Geometry: final body of the model. Coordinates: model frame, mm. Face numbers are marked on the shaded views. Round coordinates to 2 decimals unless told otherwise and drop trailing zeros. Order: outer loops, then holes, each group sorted by start corner. A loop starts at its lowest first (then second) coordinate and runs counter-clockwise, first axis right, second up. Notation, with made-up numbers: (64.5, 14.25) - (93.5, 14.25) arc R19 ccw to (93.5, 37.25) - close; hole circle Ø4 at (31, 22.5). An arc over 180 degrees is marked (long way). Put each result on its own line as item: value. Start each with the question number.
(1) Section C-C (z = 0). Output: boundary loops of the cut face in (x, y) (1 decimal), and give its area (3 significant figures).
(2) Pin query (flat end, axial travel): P1, Ø3, axis at x = 0, z = 0, coming from the -Y side (3 decimals); P2, Ø1, axis at y = 3.5, z = -2, coming from the -X side. Return the tip coordinate at first contact, or that it passes through.
(3) Pull-direction query (X, two-part tool) for the marked faces 1, 2, 3 and 4; classes: released by +X, released by -X, zero draft, split by the parting line, or undercut.
(4) Section A-A (y = 2). Output: boundary loops of the cut face in (x, z).
(5) Section B-B (x = 0). Output: boundary loops of the cut face in (y, z) (3 decimals), and give its area (3 significant figures).
(6) Material intervals for L1, parallel to Z at x = 0, y = 2.75; L2, parallel to Z at x = -1, y = 3.25; L3, parallel to Y at x = 1, z = -0.75 (3 decimals), sorted ascending. Write a range as [from, to].
from build123d import *

# Parameters (mm, degrees)
BOSS_EXTRUDE1_DEPTH = 8.255
FILLET1_R           = 0.635
SKETCH2_R           = 1.778
CUT_EXTRUDE3_DEPTH  = 6.985


with BuildPart() as part:
    # Sketch1 → Boss-Extrude1 (new body)
    with BuildSketch(Plane(origin=(0, 0, 0), x_dir=(1, 0, 0), z_dir=(0, 1, 0))):
        with BuildLine():
            Line((-3.4925, 3.048), (3.4925, 3.048))
            ThreePointArc((3.4925, 3.048), (6.5405, 0), (3.4925, -3.048))
            Line((3.4925, -3.048), (-3.4925, -3.048))
            ThreePointArc((-3.4925, -3.048), (-6.5405, 0), (-3.4925, 3.048))
        make_face()
    extrude(amount=BOSS_EXTRUDE1_DEPTH)

    # Fillet1
    fillet1_edges = [part.edges().sort_by_distance(p)[0] for p in [
        (6.5405, 8.255, 0),
        (0, 8.255, -3.048),
        (-6.5405, 8.255, 0),
        (0, 8.255, 3.048),
    ]]
    fillet(fillet1_edges, radius=FILLET1_R)

    # Sketch2 → Cut-Extrude3 (cut)
    with BuildSketch(Plane.XZ):
        Circle(SKETCH2_R)
    extrude(amount=-CUT_EXTRUDE3_DEPTH, mode=Mode.SUBTRACT)


solid = part.part
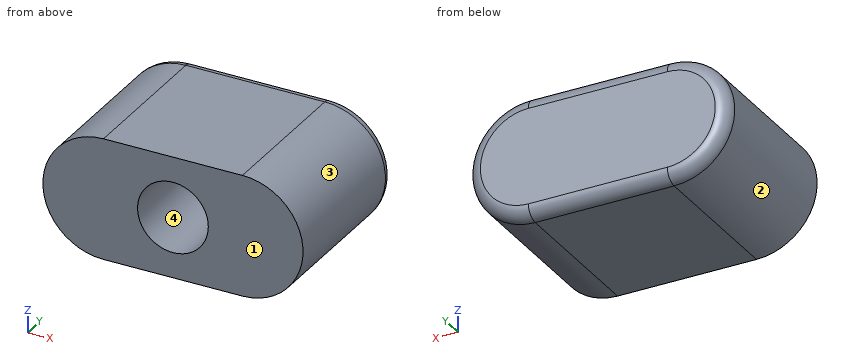
Checks:
1. outline: (-6.5, 0) - (-1.8, 0) - (-1.8, 7) - (1.8, 7) - (1.8, 0) - (6.5, 0) - (6.5, 7.6) arc R0.6 ccw to (5.9, 8.3) - (-5.9, 8.3) arc R0.6 ccw to (-6.5, 7.6) - close
1. area: 83.0 mm²
2. P1: stops at y = 6.985
2. P2: stops at x = -6.15
3. face 1: zero draft
3. face 2: released by -X
3. face 3: released by +X
3. face 4: undercut
4. outline: (-3.49, -3.05) - (3.49, -3.05) arc R3.05 ccw to (3.49, 3.05) - (-3.49, 3.05) arc R3.05 ccw to start; hole circle Ø3.56 at (0, 0)
5. outline: (0, -3.048) - (7.62, -3.048) arc R0.635 ccw to (8.255, -2.413) - (8.255, 2.413) arc R0.635 ccw to (7.62, 3.048) - (0, 3.048) - (0, 1.778) - (6.985, 1.778) - (6.985, -1.778) - (0, -1.778) - close
5. area: 25.3 mm²
6. L1: z = [-3.05, -1.78], [1.78, 3.05]
6. L2: z = [-3.05, -1.47], [1.47, 3.05]
6. L3: y = [6.985, 8.255]
